Can you work these out from the model? Positions are in its coordinate system, mm. Face numbers are marked on the shaded views. A direction names the side the tool comes from. Give positions to 0.01 mm unless a question says otherwise; leave off trailing zeros. Loops run counter-clockwise (first coordinate to the right, second up) from the corner with the lowest first, then second, coordinate; pieces in that order, holes last. Notation, with made-up numbers: M 77.5,51.5 L 98.5,51.5 A27 cw 98.5,89.5 Z; hole C 82.5,3.5 d8. An arc over 180 degrees is marked long. Answer as a JSON object with one key per item and string values.
```python
from build123d import *

# Parameters (mm, degrees)
SKETCH1_W             = 10
SKETCH1_H             = 13.75
SKETCH1_R             = 2.75
BOSS_EXTRUDE1_DEPTH   = 6
BOSS_EXTRUDE1_2_DEPTH = 6
SKETCH1_3_W           = 10
SKETCH1_3_H           = 14.5
BOSS_EXTRUDE2_DEPTH   = 32.8
SKETCH2_R             = 4
CUT_EXTRUDE1_DEPTH    = 32.8


with BuildPart() as part:
    # Sketch1 → Boss-Extrude1 (new body)
    with BuildSketch(Plane(origin=(0, 0, 0), x_dir=(1, 0, 0), z_dir=(0, 1, 0))):
        with Locations((0, 14.125)):
            Rectangle(SKETCH1_W, SKETCH1_H)
        with Locations((0, 16)):
            Circle(SKETCH1_R, mode=Mode.SUBTRACT)
    extrude(amount=BOSS_EXTRUDE1_DEPTH)



with BuildPart() as body_2:
    # Sketch1 → Boss-Extrude1 2 (new body)
    with BuildSketch(Plane(origin=(0, 0, 0), x_dir=(1, 0, 0), z_dir=(0, 1, 0))):
        with Locations((0, -14.125)):
            Rectangle(SKETCH1_W, SKETCH1_H)
        with Locations((0, -16)):
            Circle(SKETCH1_R, mode=Mode.SUBTRACT)
    extrude(amount=BOSS_EXTRUDE1_2_DEPTH)


with BuildPart() as part_1:
    add(part.part)

    add(body_2.part)  # Boss-Extrude2 merges body 2
    # Sketch1<3> → Boss-Extrude2 (add)
    with BuildSketch(Plane(origin=(0, 0, 0), x_dir=(1, 0, 0), z_dir=(0, 1, 0))):
        Rectangle(SKETCH1_3_W, SKETCH1_3_H)
    extrude(amount=BOSS_EXTRUDE2_DEPTH)

    # Sketch2 → Cut-Extrude1 (cut)
    with BuildSketch(Plane(origin=(5, 0, 0), x_dir=(0, 0, -1), z_dir=(1, 0, 0))):
        with Locations((0, 21.854969952)):
            Circle(SKETCH2_R)
    extrude(amount=-CUT_EXTRUDE1_DEPTH, mode=Mode.SUBTRACT)


solid = part_1.part
```
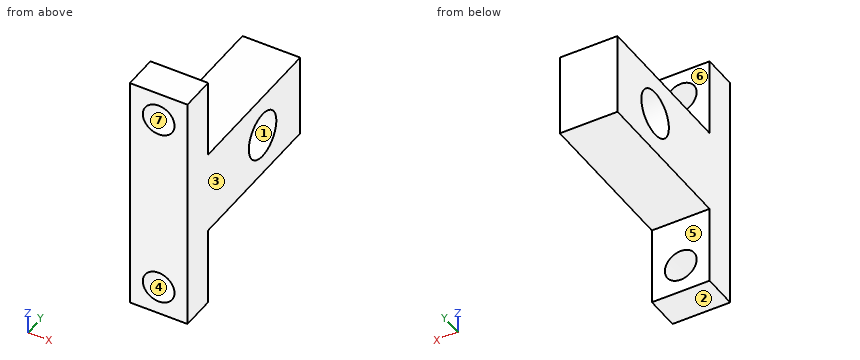
1) If we mould it in two halves opening along Z, with no side actions, what happens to the marked faces 1, 2, 3 and 4? For each: +Z half, -Z half, draft (parallel to the pull), parting line (faces both ways), or undercut.
Answer list:
{"face 1": "undercut", "face 2": "-Z half", "face 3": "draft", "face 4": "undercut"}
2) Suppose I cut it at A-A, the plane z = -16. Write out the boundary of the cut face in (x, y), and give its area (3 significant figures).
Answer list:
{"outline": "M -5,0 L -2.75,0 L -2.75,6 L -5,6 Z; M 2.75,0 L 5,0 L 5,6 L 2.75,6 Z", "area": "27.0 mm^2"}
3) Suppose I cut it at B-B, the plane x = 2. Write out the boundary of the cut face in (y, z).
Answer list:
{"outline": "M 0,-21 L 6,-21 L 6,-17.89 L 0,-17.89 Z; M 0,-14.11 L 6,-14.11 L 6,-7.25 L 32.8,-7.25 L 32.8,7.25 L 6,7.25 L 6,14.11 L 0,14.11 Z; M 0,17.89 L 6,17.89 L 6,21 L 0,21 Z; hole C 21.85,0 d8"}
4) Please list where these lines run through material, in increasing order: line 1 along Z through (x, y) = (0, 1.4); line 2 along Y through (x, z) = (-2, 0); line 3 along Z through (x, y) = (0.5, 14). Write a range as from..to.
Answer list:
{"line 1": "-21..-18.75, -13.25..13.25, 18.75..21", "line 2": "0..17.85, 25.85..32.8", "line 3": "-7.25..7.25"}
5) Suppose I cut it at C-C, the plane y = 23.5. Write out the boundary of the cut face in (x, z), and give its area (3 significant figures).
Answer list:
{"outline": "M -5,-7.25 L 5,-7.25 L 5,-3.65 L -5,-3.65 Z; M -5,3.65 L 5,3.65 L 5,7.25 L -5,7.25 Z", "area": "72.1 mm^2"}
6) For the marked faces 5, 6 and 7, which set-ups out of +Z, -Z, +X, -X, +Y, -Y let a thin tool reach every point of the face, with its end or its side?
Answer list:
{"face 5": "-Z, +X, -X, +Y", "face 6": "+Z, +X, -X, +Y", "face 7": "+Y, -Y"}
7) Will these pins go through, and if not, where does the flat tip stop? pin 1 Ø5 at (x, y) = (0.5, 21) entering from -Z; pin 2 Ø4.5 at (x, z) = (0, 16) entering from -Y.
Answer list:
{"pin 1": "z = -7.25", "pin 2": "through"}
8) Suppose I cut it at D-D, the plane y = 2. Write out the boundary of the cut face in (x, z).
Answer list:
{"outline": "M -5,-21 L 5,-21 L 5,21 L -5,21 Z; hole C 0,-16 d5.5; hole C 0,16 d5.5"}
